Here's how the part is built. I have some questions about the finished solid (model axes, mm). A direction names the side the tool comes from. Round coordinates to 2 decimals unless told otherwise and drop trailing zeros. Write each loop counter-clockwise with the first axis right and the second up, starting at its lowest first coordinate (ties: lowest second). Pieces come first, ordered by that corner, then holes. Notation, with made-up numbers: (56.25, 66) -> (99.25, 66) arc R21 cw to (99.25, 78) -> close; hole circle Ø11 at (87.5, -3). An arc over 180 degrees is marked (long way). Answer in a Markdown table with one row per item. Add a question column.
from build123d import *

# Parameters (mm, degrees)
SKIZZE1_R                       = 50
SKIZZE1_R_2                     = 5
AUFSATZ_LINEAR_AUSTRAGEN1_DEPTH = 150
SKIZZE2_W                       = 92
SKIZZE2_H                       = 50
SKIZZE2_H_2                     = 71
SCHNITT_LINEAR_AUSTRAGEN1_DEPTH = 207.155281281


with BuildPart() as part:
    # Skizze1 → Aufsatz-Linear austragen1 (new body)
    # profile 1 of 2: a face of its own
    with BuildSketch(Plane(origin=(0, 0, 0), x_dir=(0, 0, -1), z_dir=(1, 0, 0))):
        Circle(SKIZZE1_R)
        Circle(SKIZZE1_R_2, mode=Mode.SUBTRACT)
    # profile 2 of 2: a face of its own
    with BuildSketch(Plane(origin=(0, 0, 0), x_dir=(0, 0, -1), z_dir=(1, 0, 0))):
        with BuildLine():
            ThreePointArc((50, 0), (0, -50), (-50, 0))
            Line((-50, 0), (-50, -100))
            Line((-50, -100), (50, -100))
            Line((50, -100), (50, 0))
        make_face()
    extrude(amount=AUFSATZ_LINEAR_AUSTRAGEN1_DEPTH)

    # Skizze2 → Schnitt-Linear austragen1 (cut, through all)
    with BuildSketch(Plane.XY.offset(50)):
        with Locations((75, 25)):
            Rectangle(SKIZZE2_W, SKIZZE2_H)
        with Locations((75, -35.5)):
            Rectangle(SKIZZE2_W, SKIZZE2_H_2)
    extrude(amount=-SCHNITT_LINEAR_AUSTRAGEN1_DEPTH, mode=Mode.SUBTRACT)


solid = part.part
Item 1: I need wall thicknesses on line 1 along Z through (x, y) = (139.5, 0); line 2 along Y through (x, z) = (14, 0); line 3 along X through (y, z) = (-5, -5.5). Which ranges of each line are inside material? Lowest first, please. Write a range as from..to.
Item 2: If we mould it in two halves opening along Y, with no side actions, what happens to faces 1 (the cylindrical face through (14.297, 49.988, -1.099)), 2 (the flat face through (121, -11, 1)), 3 (the cylindrical face through (135.3, -4.88, 1.08)), 4 (the flat face through (74, -100, 1))? For each: pulls with the +Y half, pulls with the -Y half, needs draft (parallel to the pull), parting line crosses it, or undercut.
Item 3: If we section it at B-B on x = 135: Please give me the cut outline in (y, z), then the cut area to 3 significant figures.
Item 4: If we section it at C-C on y = 27.5: Please give me the cut outline in (x, z), then the cut area to 3 significant figures.
Item 5: For P1, Ø11.5, axis at y = 0, z = 0, coming from the -X side; P2, Ø5, axis at x = 42.5, z = -4, coming from the +Y side; P3, Ø4, axis at x = 20.5, y = 29.5, coming from the +Z side, each with a flat end and sliding along its axis, tell me the tip position at first contact or that it passes through.
Item 6: If we section it at D-D on z = -18.5: Please give me the cut outline in (x, y), then the cut area to 3 significant figures.
Item 7: On a 3-axis mill with a long thin cutter (end or side, diameter ignored), from which of +Z, -Z, +X, -X, +Y, -Y can I reach the whole of each face in a straight line? I mean faces 5 (the flat face through (74, -71, 1)), 6 (the flat face through (74, -73, -50)). Say none if no direction works.
Item 8: If we section it at A-A on z = 0: Please give me the cut outline in (x, y).
Results list:
| question | item | result |
|---|---|---|
| 1 | line 1 | -50..-5, 5..50 |
| 1 | line 2 | -100..-5, 5..50 |
| 1 | line 3 | 0..29, 121..150 |
| 2 | face 1 | pulls with the +Y half |
| 2 | face 2 | needs draft |
| 2 | face 3 | undercut |
| 2 | face 4 | pulls with the -Y half |
| 3 | outline | (-100, -50) -> (0, -50) arc R50 ccw to (0, 50) -> (-100, 50) -> close; hole circle Ø10 at (0, 0) |
| 3 | area | 13,800 mm² |
| 4 | outline | (0, -41.76) -> (29, -41.76) -> (29, 41.76) -> (0, 41.76) -> close; (121, -41.76) -> (150, -41.76) -> (150, 41.76) -> (121, 41.76) -> close |
| 4 | area | 4,840 mm² |
| 5 | P1 | x = 0 |
| 5 | P2 | y = -71 |
| 5 | P3 | z = 41.76 |
| 6 | outline | (0, -100) -> (150, -100) -> (150, 46.45) -> (121, 46.45) -> (121, -71) -> (29, -71) -> (29, 46.45) -> (0, 46.45) -> close |
| 6 | area | 11,200 mm² |
| 7 | face 5 | +Z, -Z, +Y |
| 7 | face 6 | -Z, +X, -X, +Y, -Y |
| 8 | outline | (0, -100) -> (150, -100) -> (150, -5) -> (121, -5) -> (121, -71) -> (29, -71) -> (29, -5) -> (0, -5) -> close; (0, 5) -> (29, 5) -> (29, 50) -> (0, 50) -> close; (121, 5) -> (150, 5) -> (150, 50) -> (121, 50) -> close |
